```python
from build123d import *

# Parameters (mm, degrees)
BOSS_EXTRUDE1_DEPTH = 2
SKETCH2_R           = 1.5
CUT_EXTRUDE1_DEPTH  = 162.776916151
FILLET1_R           = 2


with BuildPart() as part:
    # Sketch1 → Boss-Extrude1 (new body)
    with BuildSketch(Plane(origin=(0, 0, 0), x_dir=(1, 0, 0), z_dir=(0, 1, 0))):
        with BuildLine():
            Line((-93.626923886, -57.255296936), (-125.285208035, -62.353434177))
            ThreePointArc((-125.285208035, -62.353434177), (-139.136930256, -59.744510113), (-148.029903031, -48.8087098))
            ThreePointArc((-148.029903031, -48.8087098), (-144.651370762, -29.319378812), (-126.373822338, -21.757651079))
            Line((-126.373822338, -21.757651079), (-86.108085396, -26.140585529))
            Line((-86.108085396, -26.140585529), (-76.160414707, -32.849365164))
            Line((-76.160414707, -32.849365164), (-78.953515167, -36.996483419))
            Line((-78.953515167, -36.996483419), (-83.117646396, -37.808894096))
            Line((-83.117646396, -37.808894096), (-92.055567869, -51.079672511))
            Line((-92.055567869, -51.079672511), (-91.243157193, -55.24380374))
            Line((-91.243157193, -55.24380374), (-92.919017469, -57.732074693))
            Line((-92.919017469, -57.732074693), (-93.626923886, -57.255296936))
        make_face()
        with BuildLine():
            ThreePointArc((-128.01465119, -54.213221054), (-127.558293409, -52.505375167), (-129.266139297, -52.049017386))
            ThreePointArc((-129.266139297, -52.049017386), (-129.722497078, -53.756863273), (-128.01465119, -54.213221054))
        make_face(mode=Mode.SUBTRACT)
        with BuildLine():
            ThreePointArc((-118.499717146, -37.706675985), (-118.043359364, -35.998830097), (-119.751205252, -35.542472316))
            ThreePointArc((-119.751205252, -35.542472316), (-120.207563033, -37.250318204), (-118.499717146, -37.706675985))
        make_face(mode=Mode.SUBTRACT)
        with BuildLine():
            ThreePointArc((-137.552271527, -37.719773921), (-137.095913745, -36.011928034), (-138.803759633, -35.555570253))
            ThreePointArc((-138.803759633, -35.555570253), (-139.260117414, -37.26341614), (-137.552271527, -37.719773921))
        make_face(mode=Mode.SUBTRACT)
        with BuildLine():
            ThreePointArc((-132.903016903, -34.772829346), (-136.006249814, -46.386181381), (-124.392897779, -49.489414293))
            ThreePointArc((-124.392897779, -49.489414293), (-121.289664867, -37.876062257), (-132.903016903, -34.772829346))
        make_face(mode=Mode.SUBTRACT)
    extrude(amount=BOSS_EXTRUDE1_DEPTH)

    # Sketch2 → Cut-Extrude1 (cut, through all)
    with BuildSketch(Plane(origin=(0, 2, 0), x_dir=(1, 0, 0), z_dir=(0, 1, 0))):
        with Locations(Location((-94.319257895, -53.871812037, 0), (0, 0, 270))):
            Circle(SKETCH2_R)
        with Locations(Location((-81.035580782, -32.615630622, 0), (0, 0, 270))):
            Circle(SKETCH2_R)
        with Locations(Location((-99.81641988, -44.328419171, 0), (0, 0, 270))):
            Circle(SKETCH2_R)
        with Locations(Location((-91.026470018, -30.986543755, 0), (0, 0, 270))):
            Circle(SKETCH2_R)
    extrude(amount=-CUT_EXTRUDE1_DEPTH, mode=Mode.SUBTRACT)

    # Fillet1
    # the kernel refuses this fillet: 2 mm, written as the material it adds along each edge
    with BuildSketch(Plane(origin=(-83.117646396, 0, 37.808894096), x_dir=(-0.558620092060103, 0, 0.8294236509448968), z_dir=(0, 1, 0)), Plane(origin=(-92.055567869, 0, 51.079672511), x_dir=(0.191487032856868, 0, 0.9814951432623968), z_dir=(0, 1, 0))) as fillet1_piece_1:
        with BuildLine():
            CenterArc((FILLET1_R * 0.414213562373, FILLET1_R), FILLET1_R, 225, 45)
            Line((-FILLET1_R * 0.292893218813, FILLET1_R * 0.292893218813), (0, 0))
            Line((0, 0), (FILLET1_R * 0.414213562373, 0))
        make_face()
    extrude(amount=2)
    # the kernel refuses this fillet: 2 mm, written as the material it takes off along each edge
    with BuildSketch(Plane(origin=(-76.160414707, -4.996895665, 32.849365164), x_dir=(-0.8290765545202242, 0, -0.5591351059850148), z_dir=(0, 1, 0))) as fillet1_2_piece_1:
        with BuildLine():
            CenterArc((FILLET1_R * 0.999379132971, FILLET1_R), FILLET1_R, 180.035584106, 89.964415894)
            Line((-FILLET1_R * 0.000620674171049, FILLET1_R * 0.999378940233), (0, 0))
            Line((0, 0), (FILLET1_R * 0.999379132971, 0))
        make_face()
    extrude(amount=11.99379133, mode=Mode.SUBTRACT)
    with BuildSketch(Plane(origin=(-78.953515167, -2.071067812, 36.996483419), x_dir=(0.558620092060111, 0, -0.8294236509448913), z_dir=(0, 1, 0))) as fillet1_2_piece_2:
        with BuildLine():
            CenterArc((FILLET1_R * 0.414213562373, FILLET1_R), FILLET1_R, 225, 45)
            Line((-FILLET1_R * 0.292893218813, FILLET1_R * 0.292893218813), (0, 0))
            Line((0, 0), (FILLET1_R * 0.414213562373, 0))
        make_face()
    extrude(amount=6.142135624, mode=Mode.SUBTRACT)
    with BuildSketch(Plane(origin=(-92.919017469, -4.096888539, 57.732074693), x_dir=(-0.8294236509413199, 0, -0.5586200920654141), z_dir=(0, 1, 0))) as fillet1_2_piece_3:
        with BuildLine():
            CenterArc((2, -1.638755416), FILLET1_R, 124.977451645, 55.022548355)
            Line((0, -1.638755416), (0, 0))
            Line((0, 0), (0.853491959, 0))
        make_face()
    extrude(amount=10.193777079, mode=Mode.SUBTRACT)
    with BuildSketch(Plane(origin=(-91.243157193, -2.071067812, 55.24380374), x_dir=(-0.558620092060103, 0, 0.8294236509448968), z_dir=(0, 1, 0))) as fillet1_2_piece_4:
        with BuildLine():
            CenterArc((FILLET1_R * 0.414213562373, -FILLET1_R), FILLET1_R, 90, 45)
            Line((-FILLET1_R * 0.292893218813, -FILLET1_R * 0.292893218813), (0, 0))
            Line((0, 0), (FILLET1_R * 0.414213562373, 0))
        make_face()
    extrude(amount=6.142135624, mode=Mode.SUBTRACT)


solid = part.part
```
The listing builds one solid part. Answer for the finished solid, in the listing's coordinates (mm). A direction names the side the tool comes from. Round coordinates to 2 decimals unless told otherwise and drop trailing zeros. Loops run counter-clockwise (first coordinate to the right, second up) from the corner with the lowest first, then second, coordinate; pieces in that order, holes last. Notation, with made-up numbers: (62, 62.25) - (113, 62.25) arc R20 cw to (113, 99.25) - close; hole circle Ø8 at (-3.5, 8.5). An arc over 180 degrees is marked (long way). Return JSON: item names as keys, results as strings. Group by question number.
1. Consider probe 1 along X at (y, z) = (1.8, 44); probe 2 along X at (y, z) = (0.25, 54); probe 3 along Z at (x, y) = (-122.5, 0.2). Determine where each line is inside the solid, lowest interval first.
2. The part is cut by section B-B on x = -131. Determine the outline of the cut face in (y, z), then the cut area to 3 significant figures.
3. Which of the six approach directions +Z, -Z, +X, -X, +Y, -Y give full straight-line access (tool end or side, diameter ignored) to faces 4 (the cylindrical face through (-83.02, 0.99, 37.94)), 5 (the flat face through (-91.653, 0.986, 53.144))?
4. The mould has two halves that part along Z. Classify faces 1 (the cylindrical face through (-94.253, 1.014, 52.373)), 2 (the flat face through (-81.02, 0.99, 37.4)), 3 (the cylindrical face through (-76.97, 0.99, 33.03)): pulls with the +Z half, pulls with the -Z half, needs draft (parallel to the pull), parting line crosses it, or undercut.
5. The part is cut by section D-D on y = 1.55. State how many separate pieces and enclosed holes the cut face has, then the cut area to 3 significant figures.
6. The part is cut by section A-A on z = 41.5. Determine the outline of the cut face in (x, y), then the cut area to 3 significant figures.
7. This flat-tipped pin is pushed along its axis until it touches: P1, Ø2.5, axis at x = -91.03, z = 30.99, coming from the -Y side. Where does it stop, or does it pass through?
8. The part is cut by section C-C on z = 53.5. Determine the outline of the cut face in (x, y), then the cut area to 3 significant figures.
Resolved:
{
 "1": {"probe 1": "x = -149.06 to -136.94, -120.36 to -101.28, -98.35 to -87.29", "probe 2": "x = -145.36 to -129.54, -127.74 to -95.81, -92.82 to -91.49", "probe 3": "z = 22.18 to 36.26, 48 to 61.9"},
 "2": {"outline": "(0, 21.77) - (2, 21.77) - (2, 33.96) - (0, 33.96) - close; (0, 50.3) - (2, 50.3) - (2, 62.5) - (0, 62.5) - close", "area": "48.8 mm²"},
 "3": {"face 4": "+Z, +X, +Y, -Y", "face 5": "+X, +Y, -Y"},
 "4": {"face 1": "undercut", "face 2": "pulls with the +Z half", "face 3": "parting line crosses it"},
 "5": {"separate pieces": "1", "enclosed holes": "8", "area": "1,930 mm²"},
 "6": {"outline": "(-149.14, 0) - (-137.12, 0) - (-137.12, 2) - (-149.14, 2) - close; (-120.17, 0) - (-85.6, 0) - (-85.6, 2) - (-120.17, 2) - close", "area": "93.2 mm²"},
 "7": {"P1": "passes through"},
 "8": {"outline": "(-145.71, 0) - (-129.83, 0) - (-129.83, 2) - (-145.71, 2) - close; (-127.45, 0) - (-95.77, 0) - (-95.77, 2) - (-127.45, 2) - close; (-92.87, 0) - (-91.58, 0) - (-91.58, 2) - (-92.87, 2) - close", "area": "97.7 mm²"}
}
